Work out the finished part from the listing and answer in its coordinate system (mm). A direction names the side the tool comes from. Give positions to 0.01 mm unless a question says otherwise; leave off trailing zeros. Order: outer loops, then holes, each group sorted by start corner. A loop starts at its lowest first (then second) coordinate and runs counter-clockwise, first axis right, second up. Notation, with made-up numbers: M 63,14 L 112,14 A23 cw 112,42 Z; hole C -37.5,41.5 d9. An arc over 180 degrees is marked long. One line per item, written item: value.
from build123d import *

# Parameters (mm, degrees)
ESQUISSE2_W             = 8
ESQUISSE2_H             = 4
ENL_V_MAT_EXTRU_2_DEPTH = 2
ESQUISSE3_R             = 1
ENL_V_MAT_EXTRU_3_DEPTH = 10


with BuildPart() as part:
    # Esquisse1 → Révolution1 (revolve)
    with BuildSketch(Plane.XY, mode=Mode.PRIVATE) as r_volution1_sk:
        Polygon((-30, 0), (30, 0), (30, 5), (25, 5), (20, 7), (-20, 7), (-25, 5), (-30, 5), align=None)
    revolve(r_volution1_sk.sketch.rotate(Axis((-30, 0, 0), (1, 0, 0)), 180), axis=Axis((-30, 0, 0), (1, 0, 0)))

    # Esquisse2 → Enlèv. mat.-Extru.2 (cut)
    with BuildSketch(Plane.XY.offset(7)):
        Rectangle(ESQUISSE2_W, ESQUISSE2_H)
    extrude(amount=-ENL_V_MAT_EXTRU_2_DEPTH, mode=Mode.SUBTRACT)

    # Esquisse3 → Enlèv. mat.-Extru.3 (cut)
    with BuildSketch(Plane.XY.offset(5)):
        with Locations((2.5, 0)):
            Circle(ESQUISSE3_R)
        with Locations((-2.5, 0)):
            Circle(ESQUISSE3_R)
    extrude(amount=-ENL_V_MAT_EXTRU_3_DEPTH, mode=Mode.SUBTRACT)


solid = part.part
(1) Which of the six approach directions +Z, -Z, +X, -X, +Y, -Y give full straight-line access (tool end or side, diameter ignored) to faces 4 (the flat face through (30, 0, 0)), 5 (the cylindrical face through (-28, 5, 0)), 6 (the cylindrical face through (27, 5, 0)), 7 (the flat face through (0, 0, 5))?
Findings:
face 4: +Z, -Z, +X, +Y, -Y
face 5: -X
face 6: +X
face 7: +Z
(2) Section D-D, the plane x = 9.5 is taken. Give the vertices of the cut face in (y, z).
Findings:
outline: C 0,0 d14
(3) Find the intervals of material crossed by probe 1 along Y at (x, z) = (-2.5, -0.25); probe 2 along Y at (x, z) = (2.5, 3); probe 3 along Z at (x, y) = (-5.5, -5), in increasing order. Write a range as from..to.
Findings:
probe 1: y = -7..-1, 1..7
probe 2: y = -6.32..-1, 1..6.32
probe 3: z = -4.9..4.9
(4) Determine the mould class of faces 1 (the flat face through (-3, 0, -5)), 2 (the flat face through (-30, 0, 0)), 3 (the conical face through (-24.76, -2.35, 4.52)) for opening direction Y: pulls with the +Y half, pulls with the -Y half, needs draft (parallel to the pull), parting line crosses it, or undercut.
Findings:
face 1: undercut
face 2: needs draft
face 3: parting line crosses it
(5) Section B-B, the plane y = 0 is taken. Give the vertices of the cut face in (x, z), then the cut area to 3 significant figures.
Findings:
outline: M -30,-5 L -25,-5 L -20,-7 L 20,-7 L 25,-5 L 30,-5 L 30,5 L 25,5 L 20,7 L 4,7 L 4,5 L 3.5,5 L 3.5,-5 L 1.5,-5 L 1.5,5 L -1.5,5 L -1.5,-5 L -3.5,-5 L -3.5,5 L -4,5 L -4,7 L -20,7 L -25,5 L -30,5 Z
area: 724 mm^2
(6) Section C-C, the plane x = 2.5 is taken. Give the vertices of the cut face in (y, z).
Findings:
outline: M -2,5 L -2,6.71 A7 ccw long 2,6.71 L 2,5 L 1,5 L 1,-5 L -1,-5 L -1,5 Z
(7) Given P1, Ø1.4, axis at x = -1, z = 6, coming from the +Y side; P2, Ø1.9, axis at x = 0, z = 6, coming from the -Y side; P3, Ø2, axis at x = -10.5, z = -1.5, coming from the -Y side, each flat-ended and moving along its own axis, determine where each tip first touches the part or whether it passes through.
Findings:
P1: stops at y = 4.57
P2: stops at y = -4.85
P3: stops at y = -6.98
(8) Section A-A, the plane z = 0 is taken. Give the vertices of the cut face in (x, y).
Findings:
outline: M -30,-5 L -25,-5 L -20,-7 L 20,-7 L 25,-5 L 30,-5 L 30,5 L 25,5 L 20,7 L -20,7 L -25,5 L -30,5 Z; hole C -2.5,0 d2; hole C 2.5,0 d2
